Design review of the part shown in the three views and the two pictorial views. Dimensions are in mm from the part's minimum x, y and z. Round coordinates to 2 decimals unless told otherwise and drop trailing zeros. Order: outer loops, then holes, each group sorted by start corner. A loop starts at its lowest first (then second) coordinate and runs counter-clockwise, first axis right, second up. Notation, with made-up numbers: M 46,38 L 58,38 A8 ccw 58,43 Z; hole C 73,-28 d4. An arc over 180 degrees is marked long. Use a Markdown table: item, result. Add a question column.
(1) Take a section at B-B (z = 13.5). Write out the cut boundary in (x, y).
(2) Take a section at C-C (x = 43). Write out the cut boundary in (y, z).
(3) For pin 1 (1.5 mm diameter, centred on y = 13.5, z = 15, fed in from -X); pin 2 (1 mm diameter, centred on x = 36, y = 38, fed in from +Z); pin 3 (1 mm diameter, centred on y = 7, z = 8.5, fed in from +X), all flat-tipped, find the tip position at first contact; note any pin that passes through.
(4) Take a section at A-A (y = 26.5). Write out the cut boundary in (x, z), then the cut area to 3 significant figures.
(5) To check wall thickness, follow probe 1 along X at (y, z) = (19.5, 8.25); probe 2 along X at (y, z) = (13, 20); probe 3 along Z at (x, y) = (47, 38.5) (1 decimal). State the ranges of each line that lie inside material, in increasing order. Write a range as from..to.
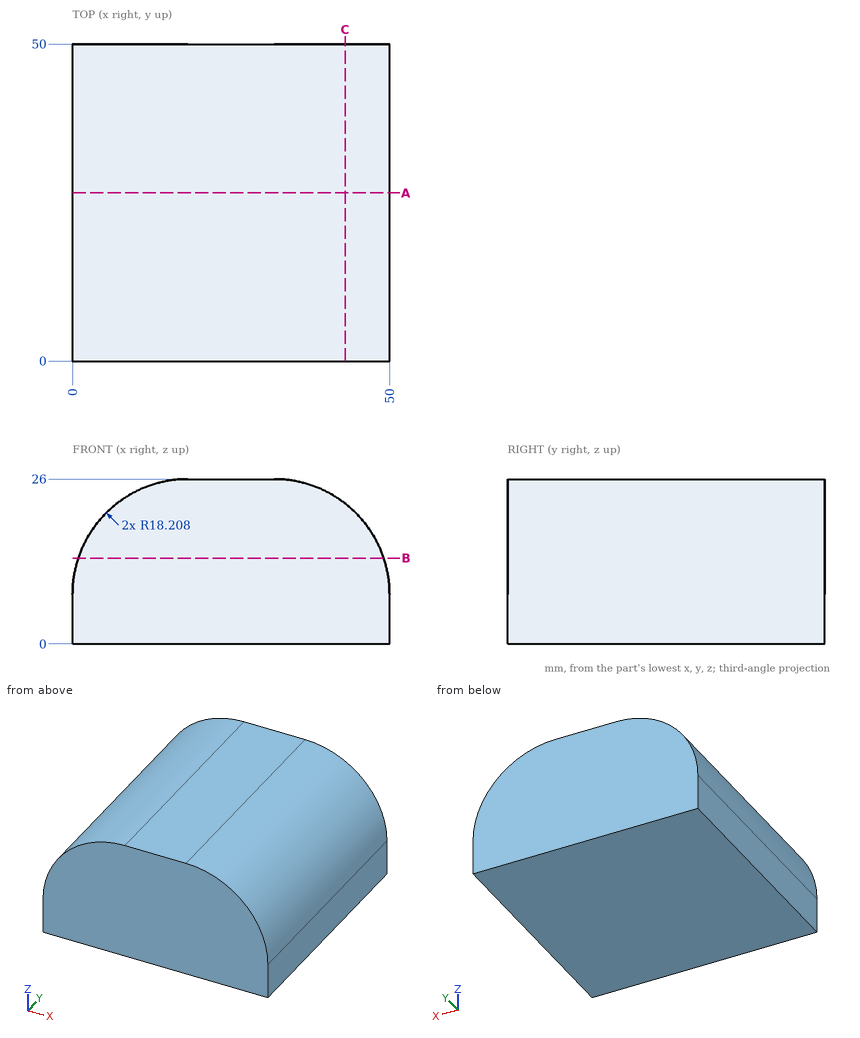
Verdict:
| question | item | result |
|---|---|---|
| 1 | outline | M 0.92,0 L 49.08,0 L 49.08,50 L 0.92,50 Z |
| 2 | outline | M 0,0 L 50,0 L 50,22.14 L 0,22.14 Z |
| 3 | pin 1 | stops at x = 1.18 |
| 3 | pin 2 | stops at z = 25.62 |
| 3 | pin 3 | stops at x = 50 |
| 4 | outline | M 0,0 L 50,0 L 50,7.79 A18.21 ccw 31.79,26 L 18.21,26 A18.21 ccw 0,7.79 Z |
| 4 | area | 1,160 mm^2 |
| 5 | probe 1 | x = 0.01..49.99 |
| 5 | probe 2 | x = 4.7..45.3 |
| 5 | probe 3 | z = 0..17.8 |
